Source: CAD feature listing. Evaluate the final solid. Frame: model axes, mm. Face numbers are marked on the shaded views. A direction names the side the tool comes from. Coordinates: 2 decimals unless noted, no trailing zeros. Write each loop counter-clockwise with the first axis right and the second up, starting at its lowest first coordinate (ties: lowest second). Pieces come first, ordered by that corner, then holes. Notation, with made-up numbers: M -2,53 L 38,53 A12 ccw 38,66 Z; hole C 17.25,33.5 d10. An arc over 180 degrees is marked long. Answer as CSV lines item,"result". Start each with the question number.
1. Contact query for flat-ended pins moving along their axis: pin 1 Ø6.5 at (x, y) = (15.5, 15.5) entering from -Z; pin 2 Ø12 at (y, z) = (8.5, -43) entering from +X; pin 3 Ø4 at (x, y) = (-15.5, 15.5) entering from +Z; pin 4 Ø5.5 at (x, z) = (-15.5, 52.5) entering from -Y. Output: stop coordinate, or through.
2. Mould query, pull axis Z, two halves, no side actions, for the marked faces 5, 6, 7 and 8. Classes: pulls with the +Z half, pulls with the -Z half, needs draft (parallel to the pull), parting line crosses it, or undercut.
3. Section A-A on z = -19. Return the cut outline in (x, y).
4. Line query: probe 1 along Z at (x, y) = (-11.5, 17); probe 2 along Z at (x, y) = (-19.5, -5); probe 3 along Z at (x, y) = (-14.5, 2.5). Output: solid intervals per line, ascending. Write a range as [from, to].
5. Reachability of the marked faces 1, 2, 3 and 4 from +Z, -Z, +X, -X, +Y, -Y: full face, straight path, thin tool, end or side. Return the list, or none.
6. Section B-B on z = -45. Return the cut outline in (x, y), plus the area to 3 significant figures.
```python
from build123d import *

# Parameters (mm, degrees)
ESBO_O1_W                                            = 40
ESBO_O1_H                                            = 100
RESSALTO_EXTRUS_O1_DEPTH                             = 20
CORTE_EXTRUS_O1_DEPTH                                = 58.445626465
CORTE_EXTRUS_O1_DEPTH_BACK                           = 40
ESBO_O2_R                                            = 16
CORTE_EXTRUS_O5_START                                = -5
ESBO_O9_W                                            = 40
ESBO_O9_H                                            = 40
CORTE_EXTRUS_O5_DEPTH                                = 35
CORTE_EXTRUS_O7_START                                = 40
ESBO_O9_4_W                                          = 40
ESBO_O9_4_H                                          = 40
CORTE_EXTRUS_O7_DEPTH                                = 35
RESSALTO_EXTRUS_O2_DEPTH                             = 6
REBAIXO_PARA_PARAFUSO_DE_M_QUINA_COM_CAB_D           = 2.4
REBAIXO_PARA_PARAFUSO_DE_M_QUINA_COM_CAB_CBORE_D     = 5
REBAIXO_PARA_PARAFUSO_DE_M_QUINA_COM_CAB_CBORE_DEPTH = 1.6
REBAIXO_PARA_PARAFUSO_DE_M_QUINA_COM_2_D             = 3.4
REBAIXO_PARA_PARAFUSO_DE_M_QUINA_COM_2_CBORE_D       = 7
REBAIXO_PARA_PARAFUSO_DE_M_QUINA_COM_2_CBORE_DEPTH   = 2.4
FILETE4_R                                            = 5
REBAIXO_PARA_PARAFUSO_DE_M_QUINA_COM_3_D             = 3.4
REBAIXO_PARA_PARAFUSO_DE_M_QUINA_COM_3_DEPTH         = 10.05
REBAIXO_PARA_PARAFUSO_DE_M_QUINA_COM_3_CBORE_D       = 7
REBAIXO_PARA_PARAFUSO_DE_M_QUINA_COM_3_CBORE_DEPTH   = 2.4
REBAIXO_PARA_PARAFUSO_DE_M_QUINA_COM_3_TIP           = 1.021463052
ESBO_O20_W                                           = 1.5
ESBO_O20_H                                           = 3
CORTE_EXTRUS_O8_DEPTH                                = 106.242576935
ESBO_O21_R                                           = 2.50059394
CORTE_EXTRUS_O9_DEPTH                                = 5
RESSALTO_EXTRUS_O3_DEPTH                             = 5
ESBO_O23_R                                           = 10
RESSALTO_EXTRUS_O4_DEPTH                             = 2
FILETE5_R                                            = 2
RESSALTO_EXTRUS_O5_START                             = -2
ESBO_O24_R                                           = 16
ESBO_O24_R_2                                         = 7.5
RESSALTO_EXTRUS_O5_DEPTH                             = 2
ESBO_O26_R                                           = 8.1
CORTE_EXTRUS_O10_DEPTH                               = 5


with BuildPart() as part:
    # Esboço1 → Ressalto-extrusão1 (new, symmetric)
    with BuildSketch(Plane(origin=(0, 0, 0), x_dir=(1, 0, 0), z_dir=(0, 1, 0))):
        Rectangle(ESBO_O1_W, ESBO_O1_H)
    extrude(amount=RESSALTO_EXTRUS_O1_DEPTH, both=True)

    # Esboço2 → Corte-extrusão1 (cut, two sides: drawn at the far end of the back side and taken through both)
    with BuildSketch(Plane.XY.offset(-CORTE_EXTRUS_O1_DEPTH_BACK)):
        Circle(ESBO_O2_R)
    extrude(amount=CORTE_EXTRUS_O1_DEPTH + CORTE_EXTRUS_O1_DEPTH_BACK, mode=Mode.SUBTRACT)

    # Esboço9 → Corte-extrusão5 (cut)
    with BuildSketch(Plane.XY.offset(CORTE_EXTRUS_O5_START)):
        Rectangle(ESBO_O9_W, ESBO_O9_H)
        with BuildLine():
            Line((17.5, -17.5), (-17.5, -17.5))
            Line((-17.5, -17.5), (-17.5, 0))
            ThreePointArc((-17.5, 0), (0, 17.5), (17.5, 0))
            Line((17.5, 0), (17.5, -17.5))
        make_face(mode=Mode.SUBTRACT)
    extrude(amount=-CORTE_EXTRUS_O5_DEPTH, mode=Mode.SUBTRACT)

    # Esboço9<4> → Corte-extrusão7 (cut)
    with BuildSketch(Plane.XY.offset(CORTE_EXTRUS_O7_START)):
        Rectangle(ESBO_O9_4_W, ESBO_O9_4_H)
        with BuildLine():
            Line((17.5, -17.5), (-17.5, -17.5))
            Line((-17.5, -17.5), (-17.5, 0))
            ThreePointArc((-17.5, 0), (0, 17.5), (17.5, 0))
            Line((17.5, 0), (17.5, -17.5))
        make_face(mode=Mode.SUBTRACT)
    extrude(amount=-CORTE_EXTRUS_O7_DEPTH, mode=Mode.SUBTRACT)

    # Esboço3 → Ressalto-extrusão2 (add)
    with BuildSketch(Plane.XZ.offset(20)):
        with BuildLine():
            Line((20, 4), (20, -4))
            Line((20, -4), (22, -4))
            ThreePointArc((22, -4), (26, 0), (22, 4))
            Line((22, 4), (20, 4))
        make_face()
        with BuildLine():
            Line((-20, -4), (-22, -4))
            ThreePointArc((-22, -4), (-26, 0), (-22, 4))
            Line((-22, 4), (-20, 4))
            Line((-20, 4), (-20, -4))
        make_face()
    extrude(amount=-RESSALTO_EXTRUS_O2_DEPTH)

    # Rebaixo para parafuso de m_quina com cab (through all)
    with Locations(Plane(origin=(0, -14, 0), x_dir=(1, 0, 0), z_dir=(0, 1, 0))):
        with Locations((22.5, 0), (-22.5, 0)):
            CounterBoreHole(REBAIXO_PARA_PARAFUSO_DE_M_QUINA_COM_CAB_D / 2, REBAIXO_PARA_PARAFUSO_DE_M_QUINA_COM_CAB_CBORE_D / 2, REBAIXO_PARA_PARAFUSO_DE_M_QUINA_COM_CAB_CBORE_DEPTH)

    # Rebaixo para parafuso de m_quina com 2 (through all)
    with Locations(Plane.XY.offset(50)):
        with Locations((-15.5, 15.5), (15.5, 15.5)):
            CounterBoreHole(REBAIXO_PARA_PARAFUSO_DE_M_QUINA_COM_2_D / 2, REBAIXO_PARA_PARAFUSO_DE_M_QUINA_COM_2_CBORE_D / 2, REBAIXO_PARA_PARAFUSO_DE_M_QUINA_COM_2_CBORE_DEPTH)

    # Filete4
    filete4_edges = [part.edges().sort_by_distance(p)[0] for p in [
        (20, 20, 45),
        (-20, 20, 0),
        (20, 20, -45),
        (-20, 20, 45),
        (20, 20, 0),
        (-20, 20, -45),
    ]]
    fillet(filete4_edges, radius=FILETE4_R)

    # Rebaixo para parafuso de m_quina com 3
    with Locations(Plane(origin=(0, 0, -50), x_dir=(-1, 0, 0), z_dir=(0, 0, -1))):
        with Locations((-15.5, 15.5), (15.5, 15.5)):
            CounterBoreHole(REBAIXO_PARA_PARAFUSO_DE_M_QUINA_COM_3_D / 2, REBAIXO_PARA_PARAFUSO_DE_M_QUINA_COM_3_CBORE_D / 2, REBAIXO_PARA_PARAFUSO_DE_M_QUINA_COM_3_CBORE_DEPTH, depth=REBAIXO_PARA_PARAFUSO_DE_M_QUINA_COM_3_DEPTH)
            with Locations((0, 0, -(REBAIXO_PARA_PARAFUSO_DE_M_QUINA_COM_3_DEPTH + REBAIXO_PARA_PARAFUSO_DE_M_QUINA_COM_3_TIP / 2))):  # 118° drill point
                Cone(0, REBAIXO_PARA_PARAFUSO_DE_M_QUINA_COM_3_D / 2, REBAIXO_PARA_PARAFUSO_DE_M_QUINA_COM_3_TIP, mode=Mode.SUBTRACT)

    # Esboço20 → Corte-extrusão8 (cut, through all)
    with BuildSketch(Plane(origin=(0, 0, -50), x_dir=(-1, 0, 0), z_dir=(0, 0, -1))):
        with Locations((7.5, 20)):
            Rectangle(ESBO_O20_W, ESBO_O20_H)
        with Locations((-7.5, 20)):
            Rectangle(ESBO_O20_W, ESBO_O20_H)
    extrude(amount=-CORTE_EXTRUS_O8_DEPTH, mode=Mode.SUBTRACT)

    # Esboço21 → Corte-extrusão9 (cut)
    with BuildSketch(Plane(origin=(0, 20, 0), x_dir=(1, 0, 0), z_dir=(0, 1, 0))):
        with Locations(Location((0, -45, 0), (0, 0, 270))):
            Circle(ESBO_O21_R)
        with Locations(Location((0, 45, 0), (0, 0, 270))):
            Circle(ESBO_O21_R)
    extrude(amount=-CORTE_EXTRUS_O9_DEPTH, mode=Mode.SUBTRACT)

    # Esboço22 → Ressalto-extrusão3 (add)
    with BuildSketch(Plane(origin=(0, 0, -50), x_dir=(-1, 0, 0), z_dir=(0, 0, -1))):
        with BuildLine():
            Line((-6.5, 20), (-6.5, 11.5))
            ThreePointArc((-6.5, 11.5), (-7.964466094, 7.964466094), (-11.5, 6.5))
            Line((-11.5, 6.5), (-20, 6.5))
            Line((-20, 6.5), (-20, 4))
            Line((-20, 4), (-9.16515139, 4))
            ThreePointArc((-9.16515139, 4), (-10, 0), (-9.16515139, -4))
            Line((-9.16515139, -4), (-20, -4))
            Line((-20, -4), (-20, -6.5))
            Line((-20, -6.5), (-11.5, -6.5))
            ThreePointArc((-11.5, -6.5), (-7.964466094, -7.964466094), (-6.5, -11.5))
            Line((-6.5, -11.5), (-6.5, -20))
            Line((-6.5, -20), (-4, -20))
            Line((-4, -20), (-4, -9.16515139))
            ThreePointArc((-4, -9.16515139), (0, -10), (4, -9.16515139))
            Line((4, -9.16515139), (4, -20))
            Line((4, -20), (6.5, -20))
            Line((6.5, -20), (6.5, -11.5))
            ThreePointArc((6.5, -11.5), (7.964466094, -7.964466094), (11.5, -6.5))
            Line((11.5, -6.5), (20, -6.5))
            Line((20, -6.5), (20, -4))
            Line((20, -4), (9.16515139, -4))
            ThreePointArc((9.16515139, -4), (10, 0), (9.16515139, 4))
            Line((9.16515139, 4), (20, 4))
            Line((20, 4), (20, 6.5))
            Line((20, 6.5), (11.5, 6.5))
            ThreePointArc((11.5, 6.5), (7.964466094, 7.964466094), (6.5, 11.5))
            Line((6.5, 11.5), (6.5, 20))
            Line((6.5, 20), (4, 20))
            Line((4, 20), (4, 9.16515139))
            ThreePointArc((4, 9.16515139), (0, 10), (-4, 9.16515139))
            Line((-4, 9.16515139), (-4, 20))
            Line((-4, 20), (-6.5, 20))
        make_face()
    ressalto_extrus_o3 = extrude(amount=RESSALTO_EXTRUS_O3_DEPTH)

    # Esboço23 → Ressalto-extrusão4 (add)
    with BuildSketch(Plane(origin=(0, 0, -55), x_dir=(-1, 0, 0), z_dir=(0, 0, -1))):
        with Locations(Location((0, 0, 0), (0, 0, 156.421821522))):
            Circle(ESBO_O23_R)
    extrude(amount=RESSALTO_EXTRUS_O4_DEPTH)

    # Filete5
    filete5_edges = [part.edges().sort_by_distance(p)[0] for p in [
        (-9.16515139, -4, -57),
    ]]
    fillet(filete5_edges, radius=FILETE5_R - 0.0001)  # a hair under: the kernel refuses the full size

    # Esboço24 → Ressalto-extrusão5 (add)
    with BuildSketch(Plane.XY.offset(50).offset(RESSALTO_EXTRUS_O5_START)):
        Circle(ESBO_O24_R)
        Circle(ESBO_O24_R_2, mode=Mode.SUBTRACT)
    extrude(amount=RESSALTO_EXTRUS_O5_DEPTH)

    # Espelhar1: Ressalto-extrusão3 across plane
    add(ressalto_extrus_o3.mirror(Plane.XY))

    # Esboço26 → Corte-extrusão10 (cut)
    with BuildSketch(Plane.XY.offset(55)):
        Circle(ESBO_O26_R)
    extrude(amount=-CORTE_EXTRUS_O10_DEPTH, mode=Mode.SUBTRACT)


solid = part.part
```
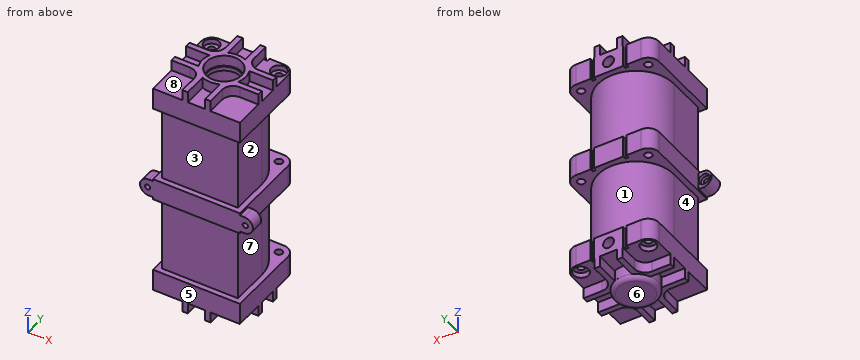
Values:
1,pin 1,"z = -47.6"
1,pin 2,"x = 20"
1,pin 3,"z = 47.6"
1,pin 4,"y = -20"
2,face 5,"needs draft"
2,face 6,"pulls with the -Z half"
2,face 7,"undercut"
2,face 8,"pulls with the +Z half"
3,outline,"M -17.5,-17.5 L 17.5,-17.5 L 17.5,0 A17.5 ccw -17.5,0 Z; hole C 0,0 d32"
4,probe 1,"[-50, -40], [-5, 5], [40, 50]"
4,probe 2,"[-55, -40], [-5, 5], [40, 55]"
4,probe 3,"[-50, -40], [48, 50]"
5,face 1,"+Y"
5,face 2,"+X, +Y, -Y"
5,face 3,"+X, -X, -Y"
5,face 4,"-X, +Y, -Y"
6,outline,"M -20,-20 L 20,-20 L 20,15 A5 ccw 15,20 L 8.25,20 L 8.25,18.5 L 6.75,18.5 L 6.75,20 L 2.5,20 L 2.5,15 L -2.5,15 L -2.5,20 L -6.75,20 L -6.75,18.5 L -8.25,18.5 L -8.25,20 L -15,20 A5 ccw -20,15 Z; hole C -15.5,15.5 d3.4; hole C 15.5,15.5 d3.4"
6,area,"1,540 mm²"
